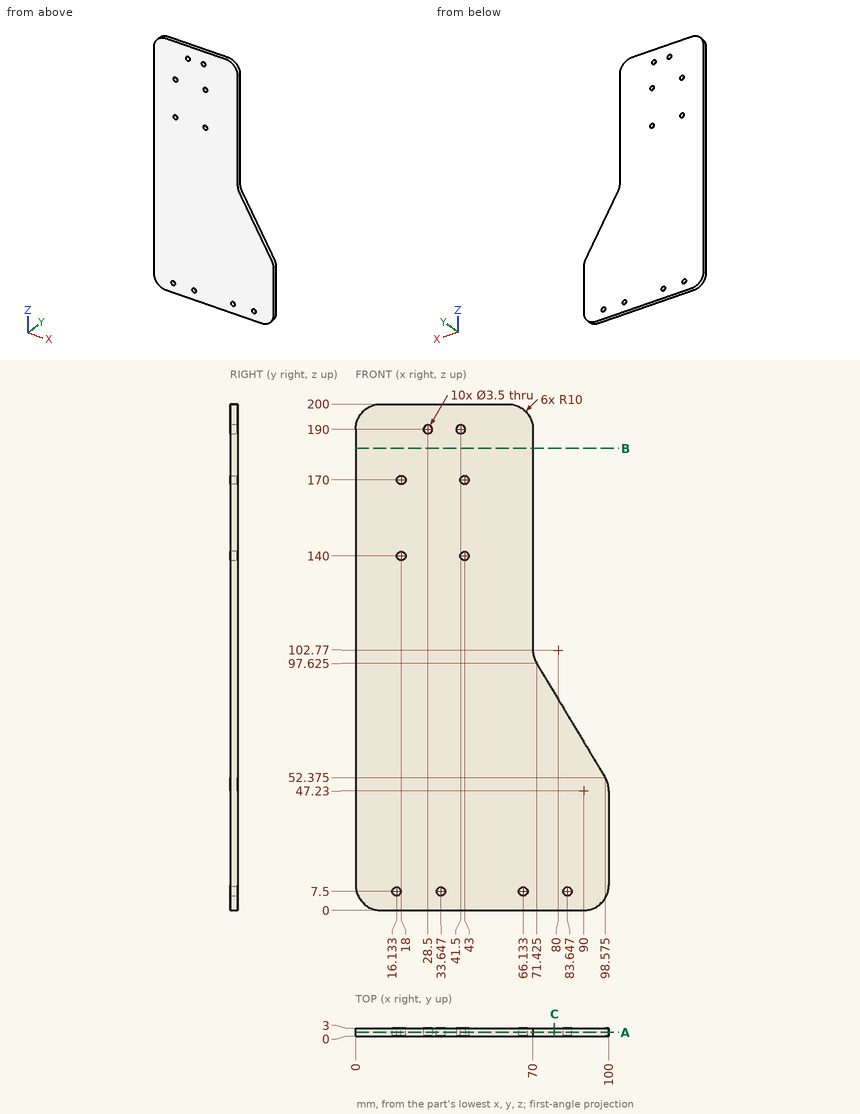
Check sheet for the drawn part. Datum: minimum x, y, z corner. Units: mm. Coordinates: 2 decimals unless noted, no trailing zeros. Write each loop counter-clockwise with the first axis right and the second up, starting at its lowest first coordinate (ties: lowest second). Pieces come first, ordered by that corner, then holes. Notation, with made-up numbers: (83, 38.5) - (120, 38.5) arc R33 cw to (120, 71.5) - close; hole circle Ø2 at (54, 29.5). An arc over 180 degrees is marked (long way). Answer as a JSON object with one key per item and string values.
(1) Cross-section at C-C on x = 78.5. Record the cut outline in (y, z).
Report:
{"outline": "(0, 0) - (3, 0) - (3, 85.83) - (0, 85.83) - close"}
(2) Thickness scan on line 1 along X through (y, z) = (0.95, 170); line 2 along X through (y, z) = (1.9, 7.5); line 3 along X through (y, z) = (2.55, 158). Record the ranges inside material, lowest first.
Report:
{"line 1": "0 to 16.25, 19.75 to 41.25, 44.75 to 70", "line 2": "0.32 to 14.38, 17.88 to 31.9, 35.4 to 64.38, 67.88 to 81.9, 85.4 to 99.68", "line 3": "0 to 70"}
(3) Cross-section at B-B on z = 182.5. Record the cut outline in (x, y), plus the area to 3 significant figures.
Report:
{"outline": "(0, 0) - (70, 0) - (70, 3) - (0, 3) - close", "area": "210 mm^2"}
(4) Cross-section at A-A on y = 1.4. Give the number of separate pieces and of enclosed holes in the cut face, plus the area to 3 significant figures.
Report:
{"separate pieces": "1", "enclosed holes": "10", "area": "16,100 mm^2"}
(5) Gauge pin test, flat ends, axial feed: pin 1 Ø3 at (x, z) = (18, 170) entering from -Y; pin 2 Ø1.5 at (y, z) = (1.5, 87.5) entering from +X; pin 3 Ø1 at (y, z) = (1.5, 49.5) entering from +X. Record the tip position at first contact, or that the pin passes through.
Report:
{"pin 1": "through", "pin 2": "x = 77.95", "pin 3": "x = 99.84"}
